Autodesk Inventor part; units mm, degrees
ref_plane "YZ Plane" through (0, 0, 0) normal (1, 0, 0) x (0, 1, 0)
ref_plane "XZ Plane" through (0, 0, 0) normal (0, 1, 0) x (-1, 0, 0)
ref_plane "XY Plane" through (0, 0, 0) normal (0, 0, 1) x (1, 0, 0)
sketch "Esboço1" plane through (0, 0, 0) normal (0, 1, 0) x (-1, 0, 0)
  circle A0 centre (0, 0) radius 30
  line L0 (29.2563, 6.6384) -> (1.1855, 6.6384)
  line L1 (1.1855, 6.6384) -> (-12.4256, 27.3058)
  line L2 (-22.8619, 19.4251) -> (-7.7387, -0.1879)
  line L3 (29.9994, -0.1879) -> (-29.9994, -0.1879) construction
  line L4 (29.2563, -7.0142) -> (1.1855, -7.0142)
  line L5 (1.1855, -7.0142) -> (-12.4256, -27.6816)
  line L6 (-22.8619, -19.8009) -> (-7.7387, -0.1879)
  point P0 (29.2563, -6.6384)
  point P1 (-23.0884, -19.1553)
  point P2 (-22.7094, -19.6031)
  point P3 (29.1685, -7.0142)
  point P4 (-12.2347, -27.3918)
  dimension "d0" = 60
extrude "Extrusão1" add sketch "Esboço1" along normal blind 42 contours A0 L4 L5 L6 L2 L1 L0
sketch "Esboço2" plane through (0, 42, 0) normal (0, 1, 0) x (1, 0, 0)
  circle A0 centre (0, 0) radius 50
  dimension "d3" = 100
extrude "Extrusão2" add sketch "Esboço2" along normal blind 2
chamfer "Chanfro1" distance 2 angle 45 3 edges at (-1.1855, 21, -7.0142) (-1.1855, 21, 6.6384) (7.7387, 21, -0.1879)
sketch "Esboço3" plane through (12.2347, 0, -27.3918) normal (-0.8352, 0, -0.55) x (-0.55, 0, 0.8352)
  line L0 (23.1979, 0) -> (0.7435, 0)
  line L1 (79.6057, 44) -> (-20.3943, 44)
  point P0 (29.6057, 0)
  dimension "d10" = 44
Geometry: final body of the model. Coordinates: model frame, mm. A direction names the side the tool comes from. Coordinates: 2 decimals unless noted, no trailing zeros. Order: outer loops, then holes, each group sorted by start corner. A loop starts at its lowest first (then second) coordinate and runs counter-clockwise, first axis right, second up. Notation, with made-up numbers: (27.25, -17) - (76.25, -17) arc R25 cw to (76.25, -4) - close; hole circle Ø2 at (39, -39.5). An arc over 180 degrees is marked (long way). Write each question's results on one line, items separated by ' | '.
(1) Section query D-D, the plane x = -39.5. Return the cut outline in (y, z).
Values found:
outline: (42, -30.66) - (44, -30.66) - (44, 30.66) - (42, 30.66) - close
(2) Line query: line 1 (Z direction, x = -7.5, y = 25); line 2 (Y direction, x = -7, z = 38); line 3 (X direction, y = 7, z = 14). Output: solid intervals per line, ascending. Write a range as [from, to].
Values found:
line 1: z = [-7.01, 6.64] | line 2: y = [42, 44] | line 3: x = [3.66, 18.68]
(3) First-contact query: pin 1 Ø12 at (y, z) = (11, -7.5) entering from -X; pin 2 Ø12 at (y, z) = (27, 20) entering from +X; pin 3 Ø10 at (x, z) = (-34.5, -12.5) entering from -Y. Flat tips, straight axial feed; report the tip coordinate or a pass-through.
Values found:
pin 1: stops at x = -29.96 | pin 2: stops at x = 22.86 | pin 3: stops at y = 42
(4) Section query A-A, the plane z = 0. Return the cut outline in (x, y).
Values found:
outline: (-50, 42) - (-30, 42) - (-30, 0) - (8.96, 0) - (8.96, 42) - (50, 42) - (50, 44) - (-50, 44) - close
(5) Set-up query: faces 5 (the face through (-1, 42, 10)), 6 (the face through (5.99, 20.71, -17.91)), 7 (the face through (-16, 21, 6.638)), 8 (the face through (15.93, 20.71, -10.81)). Return all of +Z, -Z, +X, -X, +Y, -Y with unobstructed straight access to the full face (end or side cutting, diameter ignored); none if empty.
Values found:
face 5: -Y | face 6: -Z, -X, -Y | face 7: +Z, -X, -Y | face 8: +X, -Y
(6) Section query C-C, the plane z = 10. Return the cut outline in (x, y).
Values found:
outline: (-48.99, 42) - (1.03, 42) - (1.03, 0) - (15.59, 0) - (15.59, 42) - (48.99, 42) - (48.99, 44) - (-48.99, 44) - close
(7) Section query B-B, the plane y = 15. Return the cut outline in (x, z).
Values found:
outline: (-29.26, 6.64) arc R30 ccw to (-29.17, -7.01) - (-3.19, -7.01) - (-0.09, -8.68) - (12.23, -27.39) arc R30 ccw to (22.71, -19.6) - (8.96, -1.77) - (8.96, 1.4) - (22.86, 19.43) arc R30 ccw to (12.43, 27.31) - (-0.09, 8.31) - (-3.19, 6.64) - close
(8) Mould query, pull axis Z, two halves, no side actions, for faces 1 (the face through (-1.614, 20.706, 7.485)), 2 (the face through (-1.657, 20.706, -7.838)), 3 (the face through (47.69, 42.99, 15.02)), 4 (the face through (16.01, 20.71, 10.54)). Classes: +Z half, -Z half, draft (parallel to the pull), parting line (faces both ways), or undercut.
Values found:
face 1: +Z half | face 2: -Z half | face 3: parting line | face 4: undercut
